Source: three-view drawing plus pictorial views. Frame: mm from the lowest corner of the part. A direction names the side the tool comes from. Round coordinates to 2 decimals unless told otherwise and drop trailing zeros. Order: outer loops, then holes, each group sorted by start corner. A loop starts at its lowest first (then second) coordinate and runs counter-clockwise, first axis right, second up. Notation, with made-up numbers: M 18.5,53 L 63.5,53 A14 cw 63.5,57 Z; hole C -5.5,-7.5 d7. An arc over 180 degrees is marked long. Return JSON: item names as keys, results as strings. Group by question number.
Q1. Cut plane C-C on z = 26. Output: boundary loops of the cut face in (x, y), and give its area (3 significant figures).
Q2. Contact query for flat-ended pins moving along their axis: pin 1 (5 mm diameter, centred on y = 2, z = 39, fed in from -X); pin 2 (2 mm diameter, centred on x = 48, y = 10, fed in from +Z) (1 decimal); pin 3 (4 mm diameter, centred on y = 2, z = 30, fed in from +X). Output: stop coordinate, or through.
Q3. Access query for the marked faces 5, 6 and 7. Directions: +Z, -Z, +X, -X, +Y, -Y. A direction counts if a zero-diameter tool reaches every point of the face in a straight line with its end or side. Return the directions, or none.
Q4. Ray query, probe 1 along Z at (x, y) = (8, 3.5); probe 2 along Y at (x, z) = (59, 8.5); probe 3 along Z at (x, y) = (43.5, 5.75) (1 decimal). Return the intervals inside material, ascending.
Q5. Mould query, pull axis Z, two halves, no side actions, for the marked faces 1, 2, 3 and 4. Classes: released by +Z, released by -Z, zero draft, split by the parting line, or undercut.
Q6. Cut plane A-A on y = 9. Output: boundary loops of the cut face in (x, z).
Q7. Cut plane B-B on x = 10. Output: boundary loops of the cut face in (y, z), and give its area (3 significant figures).
Q8. Cut plane D-D on x = 64. Output: boundary loops of the cut face in (y, z) (1 decimal).
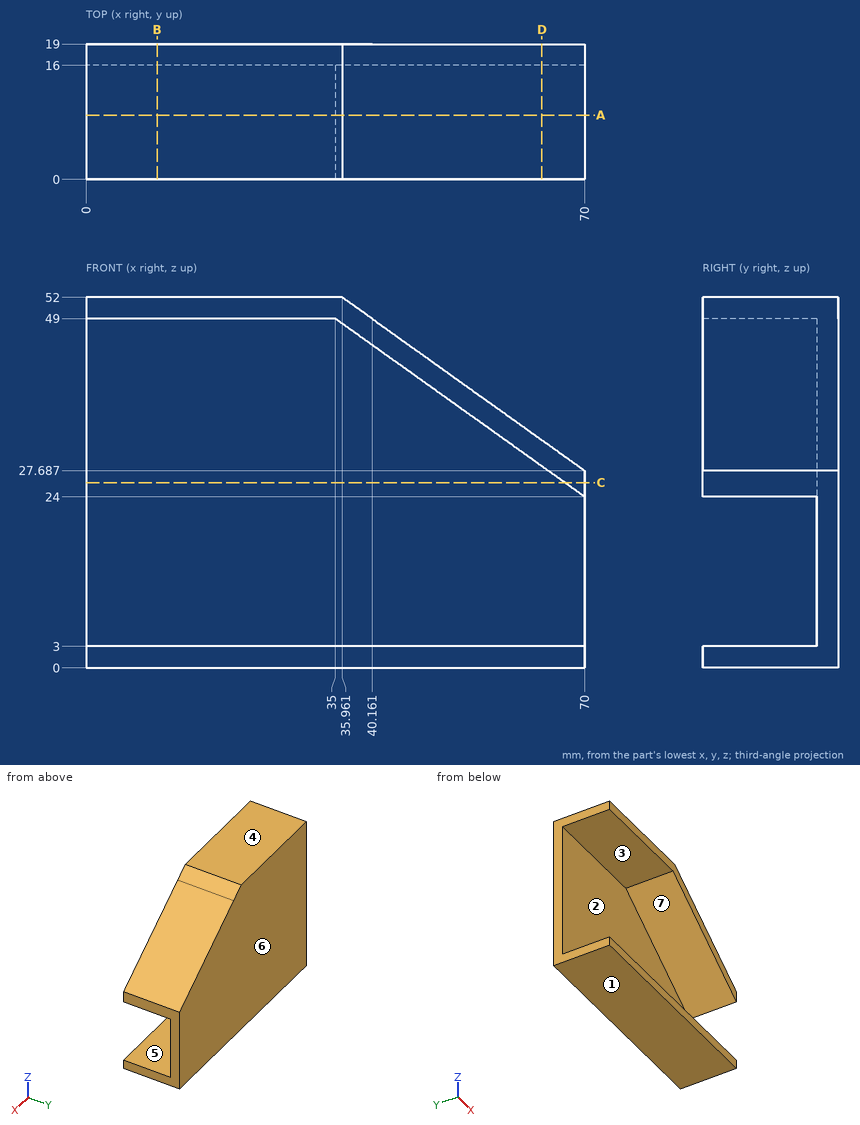
Result sheet:
{
 "1": {"outline": "M 0,16 L 67.2,16 L 67.2,0 L 70,0 L 70,19 L 0,19 Z", "area": "255 mm²"},
 "2": {"pin 1": "stops at x = 45.5", "pin 2": "stops at z = 44.1", "pin 3": "stops at x = 69.56"},
 "3": {"face 5": "+X, -X, -Y", "face 6": "+Z, -Z, +X, -X, +Y", "face 7": "-X, -Y"},
 "4": {"probe 1": "z = 0 to 3, 49 to 52", "probe 2": "y = 16 to 19", "probe 3": "z = 0 to 3, 42.9 to 46.6"},
 "5": {"face 1": "released by -Z", "face 2": "undercut", "face 3": "undercut", "face 4": "released by +Z"},
 "6": {"outline": "M 0,0 L 70,0 L 70,3 L 0,3 Z; M 0,49 L 35,49 L 70,24 L 70,27.69 L 40.16,49 L 35.96,52 L 0,52 Z"},
 "7": {"outline": "M 0,0 L 19,0 L 19,52 L 0,52 L 0,49 L 16,49 L 16,3 L 0,3 Z", "area": "252 mm²"},
 "8": {"outline": "M 0,0 L 19,0 L 19,32 L 0,32 L 0,28.3 L 16,28.3 L 16,3 L 0,3 Z"}
}
